Job drawing, mm, ordinate dimensions from the low corner. One solid piece. Round coordinates to 2 decimals unless told otherwise and drop trailing zeros. Write each loop counter-clockwise with the first axis right and the second up, starting at its lowest first coordinate (ties: lowest second). Pieces come first, ordered by that corner, then holes.
1) Saw through at B-B on y = 151. Write the cut outline in (x, z), and give its area (3 significant figures).
2) Drill centre lines: L1, parallel to Z at x = 15.5, y = 53.5; L2, parallel to Y at x = 6.75, z = 2.25 (1 decimal); L3, parallel to X at y = 210.5, z = 6.5. Where is each one in solid material? Low to high.
3) Flat gauge pins, fed straight in: pin 1 (1.5 mm diameter, centred on x = 11, z = 4, fed in from -Y); pin 2 (5 mm diameter, centred on y = 214.22, z = 5.08, fed in from +X); pin 3 (5 mm diameter, centred on y = 216.5, z = 3, fed in from -X); pin 4 (3 mm diameter, centred on y = 31.75, z = 5.08, fed in from -X). Where does each tip first touch, or does it go through?
4) Saw through at A-A on x = 6.25. Count the separate pieces of the cut face and the enclosed holes in it, and give its area (3 significant figures).
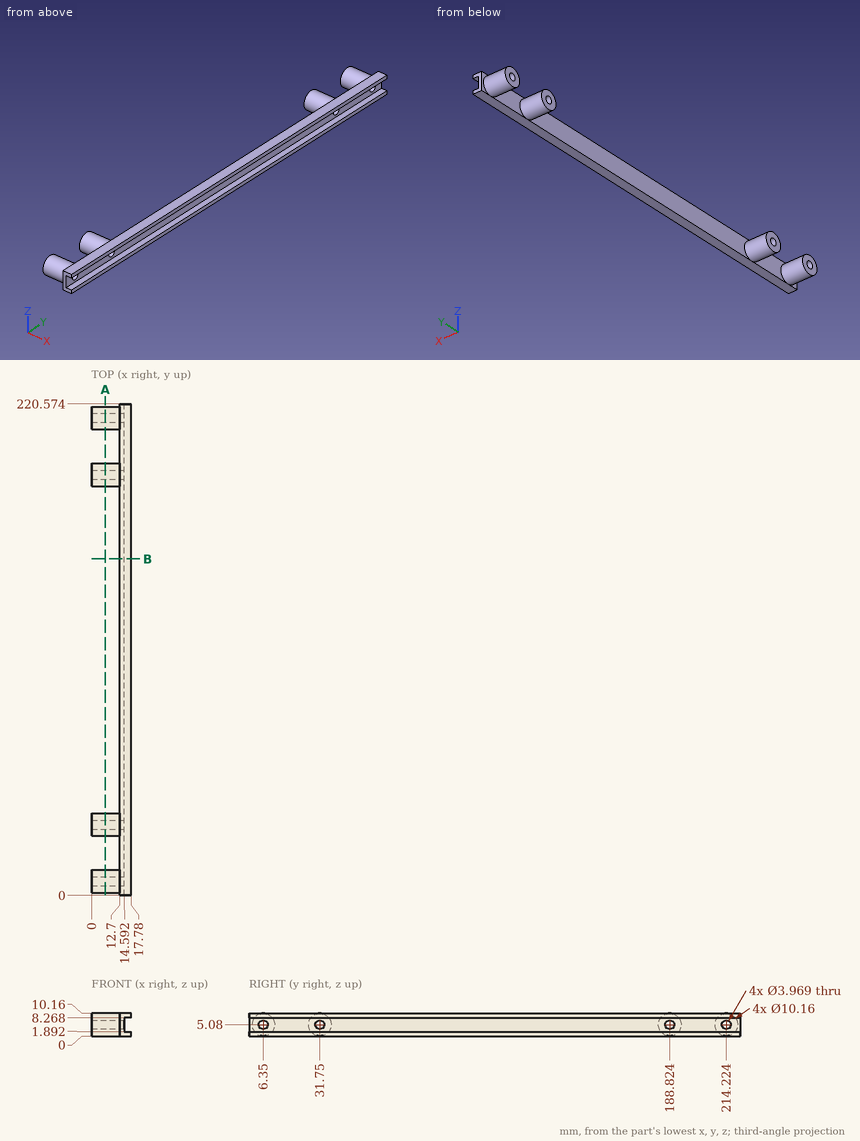
Completed:
1. outline: (12.7, 0) - (17.78, 0) - (17.78, 1.89) - (14.59, 1.89) - (14.59, 8.27) - (17.78, 8.27) - (17.78, 10.16) - (12.7, 10.16) - close
1. area: 31.3 mm2
2. L1: z = 0 to 1.89, 8.27 to 10.16
2. L2: y = 2.1 to 10.6, 27.5 to 36, 184.6 to 193, 210 to 218.4
2. L3: x = 0 to 14.59
3. pin 1: stops at y = 1.28
3. pin 2: stops at x = 14.59
3. pin 3: stops at x = 0
3. pin 4: passes through
4. separate pieces: 4
4. enclosed holes: 4
4. area: 275 mm2
